from build123d import *

# Parameters (mm, degrees)
SKETCH_1_W             = 150
SKETCH_1_H             = 110
EXTRUDE_1_DEPTH        = 5
CUT_EXTRUDE_1_REACH    = 95.14
SKETCH_2_R             = 1.5
PATTERN_LINEAR_1_COUNT = 5
PATTERN_LINEAR_1_PITCH = 21
CUT_EXTRUDE_2_REACH    = 95.14
SKETCH_3_R             = 2.5
CUT_EXTRUDE_3_REACH    = 95.14
SKETCH_4_R             = 2.5


with BuildPart() as part:
    # Sketch 1 → Extrude 1 (new body)
    with BuildSketch(Plane.XY):
        Rectangle(SKETCH_1_W, SKETCH_1_H)
    extrude(amount=EXTRUDE_1_DEPTH)

    # Sketch 2 → Cut-Extrude 1 (cut, up to next)
    with BuildSketch(Plane.XY.offset(5), mode=Mode.PRIVATE) as cut_extrude_1_sk1:
        with Locations((42, -50.5)):
            Circle(SKETCH_2_R)
    cut_extrude_1_tool1 = extrude(cut_extrude_1_sk1.sketch, amount=-CUT_EXTRUDE_1_REACH, mode=Mode.PRIVATE) & part.part
    cut_extrude_1 = cut_extrude_1_tool1.solids().sort_by_distance((42, -50.5, 5))[0]
    add(cut_extrude_1, mode=Mode.SUBTRACT)

    # Pattern Linear 1: Cut-Extrude 1 ×5
    with Locations(*[(-i * PATTERN_LINEAR_1_PITCH, 0, 0) for i in range(1, PATTERN_LINEAR_1_COUNT)]):
        add(cut_extrude_1, mode=Mode.SUBTRACT)

    # Sketch 3 → Cut-Extrude 2 (cut, up to next)
    with BuildSketch(Plane.XY.offset(5), mode=Mode.PRIVATE) as cut_extrude_2_sk1:
        with Locations((-65, 3)):
            Circle(SKETCH_3_R)
    cut_extrude_2_tool1 = extrude(cut_extrude_2_sk1.sketch, amount=-CUT_EXTRUDE_2_REACH, mode=Mode.PRIVATE) & part.part
    # Sketch 3 → Cut-Extrude 2 (cut, up to next)
    with BuildSketch(Plane.XY.offset(5), mode=Mode.PRIVATE) as cut_extrude_2_sk2:
        with Locations((-47, 3)):
            Circle(SKETCH_3_R)
    cut_extrude_2_tool2 = extrude(cut_extrude_2_sk2.sketch, amount=-CUT_EXTRUDE_2_REACH, mode=Mode.PRIVATE) & part.part
    cut_extrude_2_1 = cut_extrude_2_tool1.solids().sort_by_distance((-65, 3, 5))[0]
    add(cut_extrude_2_1, mode=Mode.SUBTRACT)
    cut_extrude_2_2 = cut_extrude_2_tool2.solids().sort_by_distance((-47, 3, 5))[0]
    add(cut_extrude_2_2, mode=Mode.SUBTRACT)
    cut_extrude_2 = cut_extrude_2_1 + cut_extrude_2_2  # Cut-Extrude 2 as one shape, for the pattern or mirror that repeats it

    # Mirror 1: Cut-Extrude 2 across plane
    add(cut_extrude_2.mirror(Plane(origin=(0, 0, 0), x_dir=(0, 0, 1), z_dir=(1, 0, 0))), mode=Mode.SUBTRACT)

    # Sketch 4 → Cut-Extrude 3 (cut, up to next)
    with BuildSketch(Plane.XY.offset(5), mode=Mode.PRIVATE) as cut_extrude_3_sk1:
        with Locations((0, 45)):
            Circle(SKETCH_4_R)
    cut_extrude_3_tool1 = extrude(cut_extrude_3_sk1.sketch, amount=-CUT_EXTRUDE_3_REACH, mode=Mode.PRIVATE) & part.part
    # Sketch 4 → Cut-Extrude 3 (cut, up to next)
    with BuildSketch(Plane.XY.offset(5), mode=Mode.PRIVATE) as cut_extrude_3_sk2:
        with Locations((0, 27)):
            Circle(SKETCH_4_R)
    cut_extrude_3_tool2 = extrude(cut_extrude_3_sk2.sketch, amount=-CUT_EXTRUDE_3_REACH, mode=Mode.PRIVATE) & part.part
    add(cut_extrude_3_tool1.solids().sort_by_distance((0, 45, 5))[0], mode=Mode.SUBTRACT)
    add(cut_extrude_3_tool2.solids().sort_by_distance((0, 27, 5))[0], mode=Mode.SUBTRACT)


solid = part.part
Source: CAD feature listing. Evaluate the final solid. Frame: model axes, mm. Give positions to 0.01 mm unless a question says otherwise; leave off trailing zeros. Write each loop counter-clockwise with the first axis right and the second up, starting at its lowest first coordinate (ties: lowest second). Pieces come first, ordered by that corner, then holes. Notation, with made-up numbers: M 31,76.25 L 68,76.25 A12 cw 68,81.25 Z; hole C 25,54 d6. An arc over 180 degrees is marked long. Return JSON: item names as keys, results as strings. Group by question number.
1) Material intervals for line 1 along Y through (x, z) = (-47, 2.4); line 2 along Y through (x, z) = (42, 3.1), sorted ascending. Write a range as [from, to].
2) Cut plane B-B, the plane y = 27. Output: boundary loops of the cut face in (x, z), plus the area to 3 significant figures.
3) Pull-direction query (Y, two-part tool) for faces 1 (the face through (-1, 55, 2)), 2 (the face through (-1, 1, 0)), 3 (the face through (44.69, 2.04, 2.54)), 4 (the face through (-43.2, -51.4, 2.5)); classes: pulls with the +Y half, pulls with the -Y half, needs draft (parallel to the pull), parting line crosses it, or undercut.
4) Cut plane A-A, the plane x = 42. Output: boundary loops of the cut face in (y, z), plus the area to 3 significant figures.
Recorded:
{
 "1": {"line 1": "y = [-55, 0.5], [5.5, 55]", "line 2": "y = [-55, -52], [-49, 55]"},
 "2": {"outline": "M -75,0 L -2.5,0 L -2.5,5 L -75,5 Z; M 2.5,0 L 75,0 L 75,5 L 2.5,5 Z", "area": "725 mm²"},
 "3": {"face 1": "pulls with the +Y half", "face 2": "needs draft", "face 3": "undercut", "face 4": "undercut"},
 "4": {"outline": "M -55,0 L -52,0 L -52,5 L -55,5 Z; M -49,0 L 55,0 L 55,5 L -49,5 Z", "area": "535 mm²"}
}
